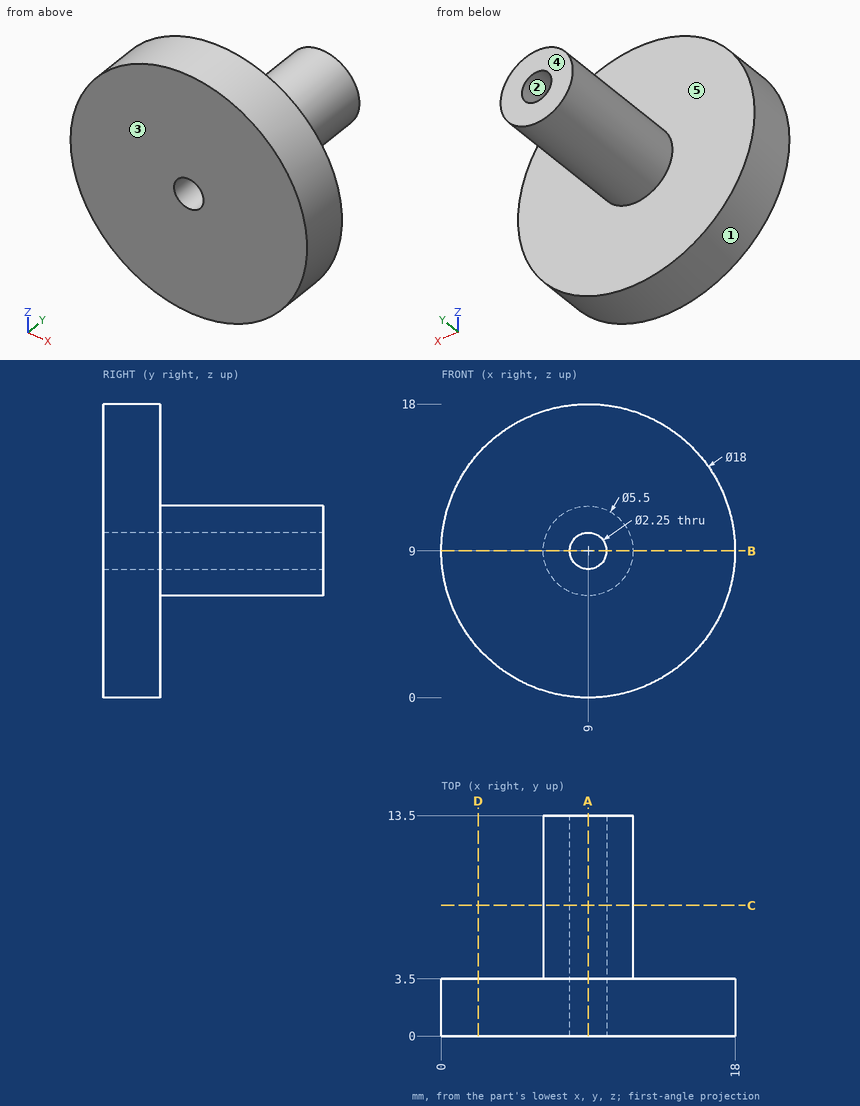
Design review of the part shown in the three views and the two pictorial views. Dimensions are in mm from the part's minimum x, y and z. A direction names the side the tool comes from. Coordinates: 2 decimals unless noted, no trailing zeros. Order: outer loops, then holes, each group sorted by start corner. A loop starts at its lowest first (then second) coordinate and runs counter-clockwise, first axis right, second up.
1) Take a section at A-A, the plane x = 9. Give the boundary of the cut face in (y, z) (3 decimals).
2) Take a section at C-C, the plane y = 8. Give the boundary of the cut face in (x, z) (3 decimals).
3) Take a section at D-D, the plane x = 2.25. Give the boundary of the cut face in (y, z), and give its area (3 significant figures).
4) Mouldability with a two-part tool opening along X and no side actions: class the marked faces 1, 2 and 3 as +X half, -X half, draft (parallel to the pull), parting line (faces both ways), or undercut.
5) Take a section at B-B, the plane z = 9. Give the boundary of the cut face in (x, y) (3 decimals).
6) Wall thickness on line 1 along Z through (x, y) = (9, 10.5) (3 decimals); line 2 along Y through (x, z) = (4, 2.5): over which ranges is each line inside the solid? List them lowest first.
7) Clearance check with flat-ended pins moving along their axes: pin 1 (8 mm diameter, centred on x = 10, z = 6, fed in from +Y); pin 2 (1 mm diameter, centred on x = 12.5, z = 2, fed in from +Y); pin 3 (1.5 mm diameter, centred on x = 15, y = 2, fed in from -Z); pin 4 (1 mm diameter, centred on x = 13, y = 3.5, fed in from -Z). State where each tip first meets the part, or that it passes through.
8) For the marked faces 4 and 5, list the 3-axis set-ups (+Z, -Z, +X, -X, +Y, -Y) from which the entire face can be reached by the end or side of a thin tool; tool diameter is ignored.
Returned:
1. outline: (0, 0) - (3.5, 0) - (3.5, 6.25) - (13.5, 6.25) - (13.5, 7.875) - (0, 7.875) - close; (0, 10.125) - (13.5, 10.125) - (13.5, 11.75) - (3.5, 11.75) - (3.5, 18) - (0, 18) - close
2. outline: circle Ø5.5 at (9, 9); hole circle Ø2.25 at (9, 9)
3. outline: (0, 3.05) - (3.5, 3.05) - (3.5, 14.95) - (0, 14.95) - close
3. area: 41.7 mm2
4. face 1: parting line
4. face 2: undercut
4. face 3: draft
5. outline: (0, 0) - (7.875, 0) - (7.875, 13.5) - (6.25, 13.5) - (6.25, 3.5) - (0, 3.5) - close; (10.125, 0) - (18, 0) - (18, 3.5) - (11.75, 3.5) - (11.75, 13.5) - (10.125, 13.5) - close
6. line 1: z = 6.25 to 7.875, 10.125 to 11.75
6. line 2: y = 0 to 3.5
7. pin 1: stops at y = 13.5
7. pin 2: stops at y = 3.5
7. pin 3: stops at z = 1.69
7. pin 4: stops at z = 0.71
8. face 4: +Z, -Z, +X, -X, +Y
8. face 5: +Y
